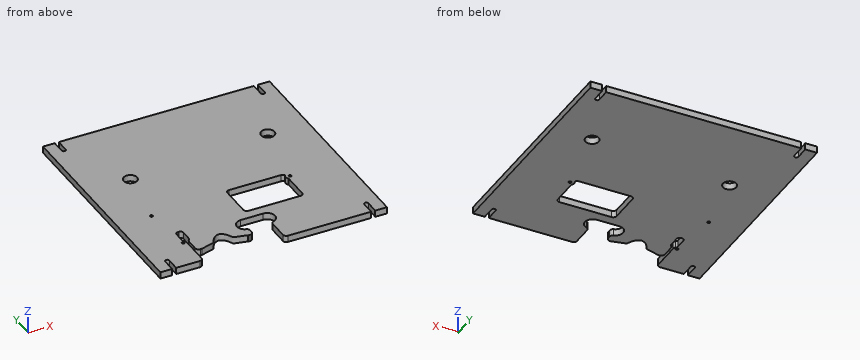
```python
from build123d import *

# Parameters (mm, degrees)
F0_R     = 2
F0_R_2   = 10
F1_DEPTH = 10


with BuildPart() as f1:
    # F0 (on Top) → F1 (new body)
    with BuildSketch(Plane.XY):
        with BuildLine():
            ThreePointArc((59.0919412169, 5.8556343452), (50.9526831397, 18.8804236674), (62.6024537054, 28.8891950556))
            Line((62.6024537054, 28.8891950556), (96.3418013123, 28.8891950556))
            ThreePointArc((96.3418013123, 28.8891950556), (107.991571878, 18.8804236674), (99.8523138008, 5.8556343452))
            ThreePointArc((99.8523138008, 5.8556343452), (97.3139335415, 4.0451239333), (96.3418013123, 1.0826450353))
            Line((96.3418013123, 1.0826450353), (96.3418013123, -3.4423905863))
            Line((96.3418013123, -3.4423905863), (96.3418013123, -28.4423905863))
            ThreePointArc((96.3418013123, -28.4423905863), (97.8062674064, -31.9779244922), (101.3418013123, -33.4423905863))
            Line((101.3418013123, -33.4423905863), (226.2431738165, -33.4423905863))
            Line((226.2431738165, -33.4423905863), (226.2431738165, -13.4423905863))
            ThreePointArc((226.2431738165, -13.4423905863), (229.2431738165, -10.4423905863), (232.2431738165, -13.4423905863))
            Line((232.2431738165, -13.4423905863), (232.2431738165, -33.4423905863))
            Line((232.2431738165, -33.4423905863), (249.8831738165, -33.4423905863))
            Line((249.8831738165, -33.4423905863), (249.8831738165, 306.5576094137))
            Line((249.8831738165, 306.5576094137), (232.2431738165, 306.5576094137))
            Line((232.2431738165, 306.5576094137), (232.2431738165, 286.5576094137))
            ThreePointArc((232.2431738165, 286.5576094137), (229.2431738165, 283.5576094137), (226.2431738165, 286.5576094137))
            Line((226.2431738165, 286.5576094137), (226.2431738165, 306.5576094137))
            Line((226.2431738165, 306.5576094137), (-66.4768261835, 306.5576094137))
            Line((-66.4768261835, 306.5576094137), (-66.4768261835, 286.5576094137))
            ThreePointArc((-66.4768261835, 286.5576094137), (-69.4768261835, 283.5576094137), (-72.4768261835, 286.5576094137))
            Line((-72.4768261835, 286.5576094137), (-72.4768261835, 306.5576094137))
            Line((-72.4768261835, 306.5576094137), (-90.1168261835, 306.5576094137))
            Line((-90.1168261835, 306.5576094137), (-90.1168261835, -33.4423905863))
            Line((-90.1168261835, -33.4423905863), (-72.4768261835, -33.4423905863))
            Line((-72.4768261835, -33.4423905863), (-72.4768261835, -13.4423905863))
            ThreePointArc((-72.4768261835, -13.4423905863), (-69.4768261835, -10.4423905863), (-66.4768261835, -13.4423905863))
            Line((-66.4768261835, -13.4423905863), (-66.4768261835, -33.4423905863))
            Line((-66.4768261835, -33.4423905863), (-30.7376475201, -33.4423905863))
            ThreePointArc((-30.7376475201, -33.4423905863), (-27.2021136142, -31.9779244922), (-25.7376475201, -28.4423905863))
            Line((-25.7376475201, -28.4423905863), (-25.7376475201, -3.4423905863))
            Line((-25.7376475201, -3.4423905863), (-25.7376475201, 14.191206688))
            ThreePointArc((-25.7376475201, 14.191206688), (-26.2085251586, 16.3094726378), (-27.5324677739, 18.0287609605))
            ThreePointArc((-27.5324677739, 18.0287609605), (-28.6705546596, 19.4817524546), (-29.1154945201, 21.2729683997))
            Line((-29.1154945201, 21.2729683997), (-29.1154945201, 37.5007453997))
            ThreePointArc((-29.1154945201, 37.5007453997), (-27.7723228668, 40.5471780201), (-24.6616755201, 41.7340793997))
            Line((-24.6616755201, 41.7340793997), (-23.4746474021, 41.7340793997))
            ThreePointArc((-23.4746474021, 41.7340793997), (-20.3442550444, 40.5612593781), (-18.9995925201, 37.5007453997))
            Line((-18.9995925201, 37.5007453997), (-18.9995925201, 21.2729683997))
            ThreePointArc((-18.9995925201, 21.2729683997), (-19.4445332952, 19.4817460524), (-20.5826230269, 18.0287486149))
            ThreePointArc((-20.5826230269, 18.0287486149), (-21.9065629195, 16.309461214), (-22.3774395201, 14.1911974832))
            Line((-22.3774395201, 14.1911974832), (-22.3774395201, -3.4423905863))
            ThreePointArc((-22.3774395201, -3.4423905863), (-20.9129734261, -6.9779244922), (-17.3774395201, -8.4423905863))
            Line((-17.3774395201, -8.4423905863), (-14.8488045963, -8.4423905863))
            add(Edge.make_bspline(
                [(-14.8488045963, -8.4423905863), (-13.8667230742, -8.0862149232), (-11.0675263436, -7.7368565701), (-9.5535565702, -6.9407787949), (-7.4752239657, -6.5093979511), (-6.0404658852, -6.1311557916), (-2.2864787406, -5.2030128278), (1.3475701923, -4.1847297196), (3.5611082397, -3.6822645324), (5.4819881536, -2.2869521331), (6.9236147383, -0.2928338043), (8.0909212332, 2.1536809326), (8.8018252555, 3.1130183139), (9.9066433173, 5.0149117757), (13.4740067588, 9.5337311578), (16.6201320308, 10.8141732124), (20.2607813027, 12.3757075827), (24.1416225167, 11.0663557699), (26.5751124317, 9.5057386468), (28.5212647481, 7.4945031555), (30.605514445, 4.8352932594), (31.5134198263, 3.0744433993), (32.6181776868, 1.1006609746), (33.5937461444, -1.0781289854), (34.6061736564, -3.5356368183), (40.2319928309, -4.632963348), (44.5783336596, -5.860680116), (49.0997891973, -6.6293952633), (53.6165002005, -7.7718986182), (54.4082808854, -8.2668507233), (54.6180656818, -8.4423905863)],
                knots=[0, 0, 0, 0, 0.0406361494, 0.0690843533, 0.0982832849, 0.1240792745, 0.1650586975, 0.2064474949, 0.237602636, 0.2688839918, 0.3023509551, 0.3363941823, 0.3586454287, 0.3892430987, 0.4390503332, 0.478234315, 0.5186842811, 0.5600640859, 0.5954673894, 0.6306059239, 0.6688365072, 0.6984296576, 0.7295419634, 0.7618620205, 0.7940667479, 0.8425634492, 0.8880772951, 0.9338149024, 0.9784648643, 1, 1, 1, 1], degree=3))
            Line((54.6180656818, -8.4423905863), (57.6024537054, -8.4423905863))
            ThreePointArc((57.6024537054, -8.4423905863), (61.1379876113, -6.9779244922), (62.6024537054, -3.4423905863))
            Line((62.6024537054, -3.4423905863), (62.6024537054, 1.0826450353))
            ThreePointArc((62.6024537054, 1.0826450353), (61.6303214762, 4.0451239333), (59.0919412169, 5.8556343452))
        make_face()
        with Locations((-30.5828261835, 15.7193741869)):
            Circle(F0_R, mode=Mode.SUBTRACT)
        with Locations((-38.5828261835, 92.2193741869)):
            Circle(F0_R, mode=Mode.SUBTRACT)
        with BuildLine():
            ThreePointArc((76.9742517439, 94.9034886555), (78.438717838, 98.4390225614), (81.9742517439, 99.9034886555))
            Line((81.9742517439, 99.9034886555), (160.1593125132, 99.9034886555))
            ThreePointArc((160.1593125132, 99.9034886555), (162.8768793148, 99.1004912382), (164.7215664672, 96.949420927))
            ThreePointArc((164.7215664672, 96.949420927), (163.2025267349, 92.3954086529), (165.1593125132, 88.0116318659))
            Line((165.1593125132, 88.0116318659), (165.1593125132, 48.6874424414))
            ThreePointArc((165.1593125132, 48.6874424414), (163.6948464191, 45.1519085355), (160.1593125132, 43.6874424414))
            Line((160.1593125132, 43.6874424414), (81.9742517439, 43.6874424414))
            ThreePointArc((81.9742517439, 43.6874424414), (78.438717838, 45.1519085355), (76.9742517439, 48.6874424414))
            Line((76.9742517439, 48.6874424414), (76.9742517439, 94.9034886555))
        make_face(mode=Mode.SUBTRACT)
        with Locations((169.8171738165, 92.7193741869)):
            Circle(F0_R, mode=Mode.SUBTRACT)
        with Locations((-22.7316567036, 183.5914050536)):
            Circle(F0_R_2, mode=Mode.SUBTRACT)
        with Locations((190.2683432964, 196.5914050536)):
            Circle(F0_R_2, mode=Mode.SUBTRACT)
    extrude(amount=F1_DEPTH)


solid = f1.part
```
Input: part model. Units: mm. Frame: model coordinates. Give positions to 0.01 mm unless a question says otherwise; leave off trailing zeros. Write each loop counter-clockwise with the first axis right and the second up, starting at its lowest first coordinate (ties: lowest second). Pieces come first, ordered by that corner, then holes. Notation, with made-up numbers: (62, -6.5) - (78, -6.5) arc R17 ccw to (78, 14.5) - close; hole circle Ø4 at (15, 87.5). An arc over 180 degrees is marked (long way). Write item = value, one per line. Start each with the question number.
1. Section query B-B, the plane y = 65. Output: boundary loops of the cut face in (x, z).
2. Section query C-C, the plane z = 7.75. Count the separate pieces of the cut face and the enclosed holes in it, then the cut area to 3 significant figures.
3. Section query A-A, the plane x = 115. Output: boundary loops of the cut face in (y, z), then the cut area to 3 significant figures.
4. First-contact query: pin 1 Ø0.9 at (x, z) = (56.5, 4.5) entering from -Y; pin 2 Ø3 at (x, z) = (84, 4) entering from -Y. Flat tips, straight axial feed; report the tip coordinate or a pass-through.
5. Ray query, L1, parallel to X at y = 65.5, z = 4; L2, parallel to Y at x = -27, z = 6.5; L3, parallel to Y at x = 154, z = 6.5. Return the intervals inside material, ascending.
Check sheet entries:
q1.outline = (-90.12, 0) - (76.97, 0) - (76.97, 10) - (-90.12, 10) - close; (165.16, 0) - (249.88, 0) - (249.88, 10) - (165.16, 10) - close
q2.separate_pieces = 1
q2.enclosed_holes = 6
q2.area = 104,000 mm2
q3.outline = (-33.44, 0) - (43.69, 0) - (43.69, 10) - (-33.44, 10) - close; (99.9, 0) - (306.56, 0) - (306.56, 10) - (99.9, 10) - close
q3.area = 2,840 mm2
q4.pin_1 = -8.44
q4.pin_2 = 28.89
q5.L1 = -90.12 to 76.97, 165.16 to 249.88
q5.L2 = -31.76 to 17.51, 41.13 to 174.55, 192.63 to 306.56
q5.L3 = -33.44 to 43.69, 99.9 to 306.56
